Source: CAD feature listing. Evaluate the final solid. Frame: model axes, mm. A direction names the side the tool comes from. Coordinates: 2 decimals unless noted, no trailing zeros. Write each loop counter-clockwise with the first axis right and the second up, starting at its lowest first coordinate (ties: lowest second). Pieces come first, ordered by that corner, then holes. Notation, with made-up numbers: (87, -23.5) -> (139, -23.5) arc R8 cw to (139, -14.5) -> close; hole circle Ø4 at (41.25, 69). An arc over 180 degrees is marked (long way). Write item = value, one per line.
from build123d import *

# Parameters (mm, degrees)
SKETCH1_R           = 1.75
BOSS_EXTRUDE1_DEPTH = 1.5
SKETCH2_R           = 14.5
BOSS_EXTRUDE2_DEPTH = 10.5
SKETCH3_R           = 11
BOSS_EXTRUDE3_DEPTH = 3
FILLET1_R           = 5
FILLET2_R           = 3


# Some blends are built 0.0001 mm under size
with BuildPart() as part:
    # Sketch1 → Boss-Extrude1 (new body)
    with BuildSketch(Plane(origin=(0, 0, 0), x_dir=(1, 0, 0), z_dir=(0, 1, 0))):
        with BuildLine():
            Line((-22.25, -4.763139721), (-9.177222982, -13.106432709))
            ThreePointArc((-9.177222982, -13.106432709), (0, -16), (9.177222982, -13.106432709))
            Line((9.177222982, -13.106432709), (22.25, -4.763139721))
            ThreePointArc((22.25, -4.763139721), (25, 0), (22.25, 4.763139721))
            Line((22.25, 4.763139721), (9.177222982, 13.106432709))
            ThreePointArc((9.177222982, 13.106432709), (0, 16), (-9.177222982, 13.106432709))
            Line((-9.177222982, 13.106432709), (-22.25, 4.763139721))
            ThreePointArc((-22.25, 4.763139721), (-25, 0), (-22.25, -4.763139721))
        make_face()
        with Locations(Location((-19.5, 0, 0), (0, 0, 270))):
            Circle(SKETCH1_R, mode=Mode.SUBTRACT)
        with Locations(Location((19.5, 0, 0), (0, 0, 270))):
            Circle(SKETCH1_R, mode=Mode.SUBTRACT)
    extrude(amount=BOSS_EXTRUDE1_DEPTH)

    # Sketch2 → Boss-Extrude2 (add)
    with BuildSketch(Plane(origin=(0, 1.5, 0), x_dir=(1, 0, 0), z_dir=(0, 1, 0))):
        with Locations(Location((0, 0, 0), (0, 0, 90))):
            Circle(SKETCH2_R)
    extrude(amount=BOSS_EXTRUDE2_DEPTH)

    # Sketch3 → Boss-Extrude3 (add)
    with BuildSketch(Plane(origin=(0, 12, 0), x_dir=(1, 0, 0), z_dir=(0, 1, 0))):
        with Locations(Location((0, 0, 0), (0, 0, 270))):
            Circle(SKETCH3_R)
    extrude(amount=BOSS_EXTRUDE3_DEPTH)

    # Sketch5 → Revolve1 (revolve)
    with BuildSketch(Plane.XY):
        with BuildLine():
            Line((0, 15), (0, 21))
            ThreePointArc((0, 21), (4.242640687, 19.242640687), (6, 15))
            Line((6, 15), (0, 15))
        make_face()
    revolve(axis=Axis((0, 15, 0), (0, 1, 0)))

    # Fillet1
    # the kernel refuses this fillet: 5 mm, written as the material it takes off along each edge
    with BuildSketch(Plane(origin=(0, 12, 0), x_dir=(0, 0, -1), z_dir=(1, 0, 0))) as fillet1_piece_1:
        with BuildLine():
            CenterArc((9.5, -4.769696007), FILLET1_R, 0, 72.542396876)
            Line((11, 0), (11.03, 0.09539392))
            ThreePointArc((11.03, 0.09539392), (12.75, 0.1), (14.5, 0.1))
            Line((14.5, 0.1), (14.6, 0))
            Line((14.6, 0), (14.6, -4.769696007))
            Line((14.6, -4.769696007), (14.5, -4.769696007))
        make_face()
    revolve(axis=Axis((0, 12, 0), (0, 1, 0)), mode=Mode.SUBTRACT)

    # Fillet2
    fillet2_edges = [part.edges().sort_by_distance(p)[0] for p in [
        (0, 15, -11),
    ]]
    fillet(fillet2_edges, radius=FILLET2_R - 0.0001)  # a hair under: the kernel refuses the full size


solid = part.part
1) First-contact query: pin 1 Ø5 at (y, z) = (6.5, -4.5) entering from +X; pin 2 Ø6 at (x, y) = (1, 11.5) entering from -Z; pin 3 Ø5 at (y, z) = (8.5, -4) entering from -X. Flat tips, straight axial feed; report the tip coordinate or a pass-through.
Answer block:
pin_1 = 14.36
pin_2 = -14.32
pin_3 = -14.39
2) Cut plane B-B, the plane x = 19.5. Output: boundary loops of the cut face in (y, z), and give its area (3 significant figures).
Answer block:
outline = (0, -6.52) -> (1.5, -6.52) -> (1.5, -1.75) -> (0, -1.75) -> close; (0, 1.75) -> (1.5, 1.75) -> (1.5, 6.52) -> (0, 6.52) -> close
area = 14.3 mm2
3) Material intervals for probe 1 along Y at (x, z) = (-16, 3.5); probe 2 along Y at (x, z) = (6.5, 4); probe 3 along X at (y, z) = (18.75, 3.5), sorted ascending. Write a range as [from, to].
Answer block:
probe_1 = [0, 1.5]
probe_2 = [0, 15]
probe_3 = [-3.11, 3.11]
4) Cut plane D-D, the plane y = 17. Output: boundary loops of the cut face in (x, z), and give its area (3 significant figures).
Answer block:
outline = circle Ø11.31 at (0, 0)
area = 101 mm2
5) Pull-direction query (X, two-part tool) for faces 1 (the flat face through (15.622, 0.74, 8.993)), 2 (the cylindrical face through (-17.765, 0.74, -0.228)), 3 (the cylindrical face through (0, 1, -16)); classes: +X half, -X half, draft (parallel to the pull), parting line (faces both ways), or undercut.
Answer block:
face_1 = +X half
face_2 = undercut
face_3 = parting line
6) Reachability of faces 4 (the cylindrical face through (0, 1, 16)), 5 (the flat face through (6, 15, -2)) from +Z, -Z, +X, -X, +Y, -Y: full face, straight path, thin tool, end or side. Return the list, or none.
Answer block:
face_4 = +Z, +Y, -Y
face_5 = +Y
7) Cut plane C-C, the plane y = 3. Output: boundary loops of the cut face in (x, z).
Answer block:
outline = circle Ø29 at (0, 0)
8) Cut plane A-A, the plane z = 0. Give the number of separate pieces and of enclosed holes in the cut face, and give its area (3 significant figures).
Answer block:
separate_pieces = 3
enclosed_holes = 0
area = 479 mm2
